```python
from build123d import *

# Parameters (mm, degrees)
F0_W     = 101.6
F0_H     = 33.02
F1_DEPTH = 4.0386
F3_DEPTH = 76.2
F4_DEPTH = 38.1
F5_DEPTH = 38.1


with BuildPart() as f1:
    # F0 (on Top) → F1 (new body)
    with BuildSketch(Plane.XY):
        Rectangle(F0_W, F0_H)
    extrude(amount=F1_DEPTH)

    # F2 (on face) → F3 (cut)
    with BuildSketch(Plane.YZ.offset(50.8)):
        Polygon((-16.51, 0), (-14.06698055, 0), (-14.06698055, 2.3274338565), (-16.51, 3.0226), align=None)
        Polygon((16.51, 0), (16.51, 3.0226), (14.06698055, 2.3274338565), (14.06698055, 0), align=None)
    extrude(amount=-F3_DEPTH, mode=Mode.SUBTRACT)

    # F4 (cut): a face of the model
    f4_faces = [f1.faces().sort_by_distance(p)[0] for p in [
        (-25.4, -15.3413966196, 1.345035768),
    ]]
    extrude(f4_faces, amount=-F4_DEPTH, mode=Mode.SUBTRACT)

    # F5 (cut): a face of the model
    f5_faces = [f1.faces().sort_by_distance(p)[0] for p in [
        (-25.4, 15.3413966196, 1.345035768),
    ]]
    extrude(f5_faces, amount=-F5_DEPTH, mode=Mode.SUBTRACT)


solid = f1.part
```
Source: CAD feature listing. Evaluate the final solid. Frame: model axes, mm. A direction names the side the tool comes from. Give positions to 0.01 mm unless a question says otherwise; leave off trailing zeros. Loops run counter-clockwise (first coordinate to the right, second up) from the corner with the lowest first, then second, coordinate; pieces in that order, holes last. Notation, with made-up numbers: (-31.5, 67.5) - (-12.5, 67.5) arc R7 cw to (-12.5, 72.5) - close; hole circle Ø9 at (39, 60.25). An arc over 180 degrees is marked (long way). Use CSV: the item, a comma, the result in double quotes. Start each with the question number.
1. Ray query, L1, parallel to Y at x = 13.5, z = 1.1. Return the intervals inside material, ascending.
2. Section B-B (z = 1.4). Output: boundary loops of the cut face in (x, y), then the cut area to 3 significant figures.
3. Section A-A (x = 39). Output: boundary loops of the cut face in (y, z).
4. Pin query (flat end, axial travel): pin 1 (2 mm diameter, centred on x = 3, z = 3, fed in from -Y); pin 2 (1.2 mm diameter, centred on x = 6, z = 1, fed in from +Y); pin 3 (0.7 mm diameter, centred on x = -19.5, z = 1.5, fed in from -Y). Return the tip coordinate at first contact, or that it passes through.
5. Reachability of faces 1 (the flat face through (1, 14.067, 1)), 2 (the flat face through (1, -14.067, 1)), 3 (the flat face through (-1, 0, 4.039)) from +Z, -Z, +X, -X, +Y, -Y: full face, straight path, thin tool, end or side. Return the list, or none.
Response:
1,L1,"-14.07 to 14.07"
2,outline,"(-50.8, -14.07) - (50.8, -14.07) - (50.8, 14.07) - (-50.8, 14.07) - close"
2,area,"2,860 mm²"
3,outline,"(-16.51, 3.02) - (-14.07, 2.33) - (-14.07, 0) - (14.07, 0) - (14.07, 2.33) - (16.51, 3.02) - (16.51, 4.04) - (-16.51, 4.04) - close"
4,pin 1,"y = -16.51"
4,pin 2,"y = 14.07"
4,pin 3,"y = -14.07"
5,face 1,"-Z, +X, -X, +Y"
5,face 2,"-Z, +X, -X, -Y"
5,face 3,"+Z, +X, -X, +Y, -Y"
